from build123d import *

# Parameters (mm, degrees)
SKETCH1_W           = 99.06
SKETCH1_H           = 360.68
BOSS_EXTRUDE1_DEPTH = 12.7
SKETCH3_W           = 32.004
SKETCH3_H           = 11.43
BOSS_EXTRUDE3_DEPTH = 20.32
SKETCH2_W           = 55.88
SKETCH2_H           = 12.7
BOSS_EXTRUDE4_DEPTH = 7.62
CUT_EXTRUDE2_DEPTH  = 38.1
SKETCH6_W           = 50.8
SKETCH6_H           = 5.08
CUT_EXTRUDE3_DEPTH  = 2.54
SKETCH7_R           = 50.8
SKETCH7_R_2         = 46.355
CUT_EXTRUDE4_DEPTH  = 366.559302576


with BuildPart() as part:
    # Sketch1 → Boss-Extrude1 (new body)
    with BuildSketch(Plane.XY):
        Rectangle(SKETCH1_W, SKETCH1_H)
    extrude(amount=BOSS_EXTRUDE1_DEPTH)

    # Sketch3 → Boss-Extrude3 (add)
    with BuildSketch(Plane(origin=(0, 0, 0), x_dir=(-1, 0, 0), z_dir=(0, 0, -1))):
        with Locations((0, -43.815)):
            Rectangle(SKETCH3_W, SKETCH3_H)
        with Locations((0, -159.385)):
            Rectangle(SKETCH3_W, SKETCH3_H)
    boss_extrude3 = extrude(amount=BOSS_EXTRUDE3_DEPTH)

    # Sketch2 → Boss-Extrude4 (add, symmetric)
    with BuildSketch(Plane.XY.offset(12.7)):
        with Locations((0, 171.45)):
            Rectangle(SKETCH2_W, SKETCH2_H)
        with Locations((0, -19.05)):
            Rectangle(SKETCH2_W, SKETCH2_H)
    extrude(amount=BOSS_EXTRUDE4_DEPTH, both=True)

    # Mirror1: Boss-Extrude3 across plane
    add(boss_extrude3.mirror(Plane.XY.offset(6.35)))

    # Sketch5 → Cut-Extrude2 (cut, symmetric)
    with BuildSketch(Plane(origin=(0, 0, 0), x_dir=(0, 0, -1), z_dir=(1, 0, 0))):
        Polygon((20.32, -153.67), (0, -165.1), (20.32, -165.1), align=None)
        Polygon((-33.02, -153.67), (-12.7, -165.1), (-33.02, -165.1), align=None)
        Polygon((-33.02, -49.53), (-33.02, -38.1), (-12.7, -38.1), align=None)
        Polygon((20.32, -49.53), (0, -38.1), (20.32, -38.1), align=None)
        Polygon((-12.7, 177.8), (-20.32, 165.1), (-20.32, 177.8), align=None)
        Polygon((-20.32, -12.7), (-12.7, -25.4), (-20.32, -25.4), align=None)
    extrude(amount=CUT_EXTRUDE2_DEPTH, both=True, mode=Mode.SUBTRACT)

    # Sketch6 → Cut-Extrude3 (cut)
    with BuildSketch(Plane(origin=(0, 180.34, 0), x_dir=(1, 0, 0), z_dir=(0, 1, 0))):
        with Locations((0, -6.35)):
            Rectangle(SKETCH6_W, SKETCH6_H)
    cut_extrude3 = extrude(amount=-CUT_EXTRUDE3_DEPTH, mode=Mode.SUBTRACT)

    # Mirror2: Cut-Extrude3 across plane
    add(cut_extrude3.mirror(Plane.ZX), mode=Mode.SUBTRACT)

    # Sketch7 → Cut-Extrude4 (cut, through all)
    with BuildSketch(Plane(origin=(0, 180.34, 0), x_dir=(1, 0, 0), z_dir=(0, 1, 0))):
        with Locations((0, -6.35)):
            Circle(SKETCH7_R)
        with Locations((0, -6.35)):
            Circle(SKETCH7_R_2, mode=Mode.SUBTRACT)
    extrude(amount=-CUT_EXTRUDE4_DEPTH, mode=Mode.SUBTRACT)


solid = part.part
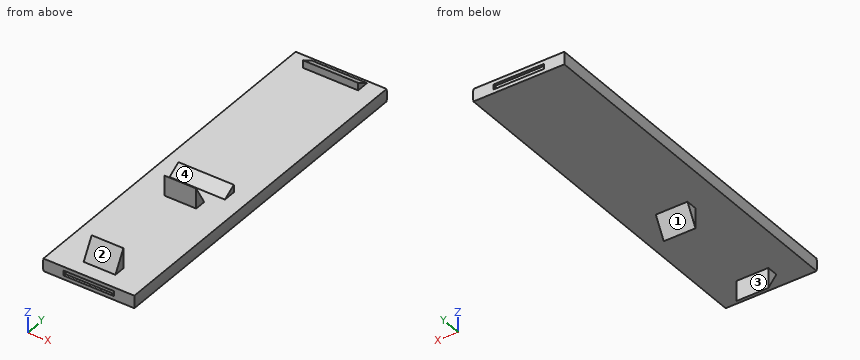
Model file for the job. Use its own axes, mm. Face numbers are marked on the shaded views. Round coordinates to 2 decimals unless told otherwise and drop trailing zeros. Loops run counter-clockwise (first coordinate to the right, second up) from the corner with the lowest first, then second, coordinate; pieces in that order, holes last.
1. Mould opens along Y. For the marked faces 1, 2, 3 and 4 say: +Y half, -Y half, draft (parallel to the pull), parting line (faces both ways), or undercut.
Check values:
face 1: +Y half
face 2: -Y half
face 3: undercut
face 4: undercut
2. Wall check: probe 1 along Y at (x, z) = (7.5, 18.5); probe 2 along Z at (x, y) = (28, -137); probe 3 along X at (y, z) = (-38.5, 4). Give the ranges that are in metal, low to high.
Check values:
probe 1: y = -161.84 to -153.67, -49.53 to -41.36, -15.73 to -12.7, 165.1 to 168.13
probe 2: z = 0 to 12.7
probe 3: x = -46.3 to 46.3
3. Drop flat-ended pins along their axis: P1, Ø12.5, axis at y = -43.5, z = -7, coming from the -X side; P2, Ø0.8, axis at x = -8.5, y = -179, coming from the -Z side; P3, Ø22.5, axis at x = 1, z = -15, coming from the -Y side. Give the stop position or say it passes through.
Check values:
P1: stops at x = -16
P2: stops at z = 0
P3: stops at y = -162.99
4. Band-saw the part on A-A, the plane z = 23.5. List the corners of the cut face in (x, y) (3 decimals), and give its area (3 significant figures).
Check values:
outline: (-16.002, -159.025) - (16.002, -159.025) - (16.002, -153.67) - (-16.002, -153.67) - close; (-16.002, -49.53) - (16.002, -49.53) - (16.002, -44.175) - (-16.002, -44.175) - close
area: 343 mm2
5. Band-saw the part on C-C, the plane y = 62.5. List the corners of the cut face in (x, z) (3 decimals), and give its area (3 significant figures).
Check values:
outline: (-45.918, 0) - (45.918, 0) arc R46.355 ccw to (45.918, 12.7) - (-45.918, 12.7) arc R46.355 ccw to start
area: 1,170 mm2
6. Band-saw the part on D-D, the plane x = 21. List the corners of the cut face in (y, z), and give its area (3 significant figures).
Check values:
outline: (-180.34, 0) - (180.34, 0) - (180.34, 3.81) - (177.8, 3.81) - (177.8, 8.89) - (180.34, 8.89) - (180.34, 12.7) - (177.8, 12.7) - (165.1, 20.32) - (165.1, 12.7) - (-12.7, 12.7) - (-12.7, 20.32) - (-25.4, 12.7) - (-180.34, 12.7) - (-180.34, 8.89) - (-177.8, 8.89) - (-177.8, 3.81) - (-180.34, 3.81) - close
area: 4,650 mm2
